from build123d import *

# Parameters (mm, degrees)
PAD017_DEPTH    = 28
SKETCH059_R     = 1.3
POCKET008_DEPTH = 48


with BuildPart() as part:
    # Sketch055 → Pad017 (new body)
    with BuildSketch(Plane.YZ):
        with BuildLine():
            ThreePointArc((0, -20.4), (17.463482, -10.544515), (18.053328, 9.499334))
            Line((18.053328, 9.499334), (23.529825, 12.66119))
            ThreePointArc((0, -26.72), (22.937583, -13.704952), (23.529825, 12.66119))
            Line((0, -20.4), (0, -26.72))
        make_face()
    extrude(amount=-PAD017_DEPTH)

    # Sketch056 → AdditiveLoft002 section 0
    with BuildSketch(Plane.YZ):
        with BuildLine():
            Line((19.650206, 5.479909), (25.72, 5.479909))
            Line((25.72, 5.479909), (25.72, -5.479909))
            Line((25.72, -5.479909), (19.650206, -5.479909))
            ThreePointArc((19.650206, -5.479909), (20.4, 0), (19.650206, 5.479909))
        make_face()
    # Sketch057 → AdditiveLoft002 section 1
    with BuildSketch(Plane.YZ.offset(17.36)):
        with BuildLine():
            Line((19.650206, 5.479909), (23.06, 5.479909))
            Line((23.06, 5.479909), (23.06, -5.479909))
            Line((23.06, -5.479909), (19.650206, -5.479909))
            ThreePointArc((19.650206, -5.479909), (20.4, 0), (19.650206, 5.479909))
        make_face()
    loft()

    # Sketch058 → Groove001 (revolve, cut)
    with BuildSketch(Plane.XY):
        Polygon((-28, 27.4), (-26, 27.4), (-26, 25.4), (-4, 25.4), (0, 27.709401), (0, 63.2), (-28, 63.2), align=None)
    revolve(axis=Axis((0, 0, 0), (1, 0, 0)), mode=Mode.SUBTRACT)

    # Sketch059 → Pocket008 (cut)
    with BuildSketch(Plane.YZ.offset(20.4)):
        with Locations((22.695, 0)):
            Circle(SKETCH059_R)
    extrude(amount=-POCKET008_DEPTH, mode=Mode.SUBTRACT)


solid = part.part
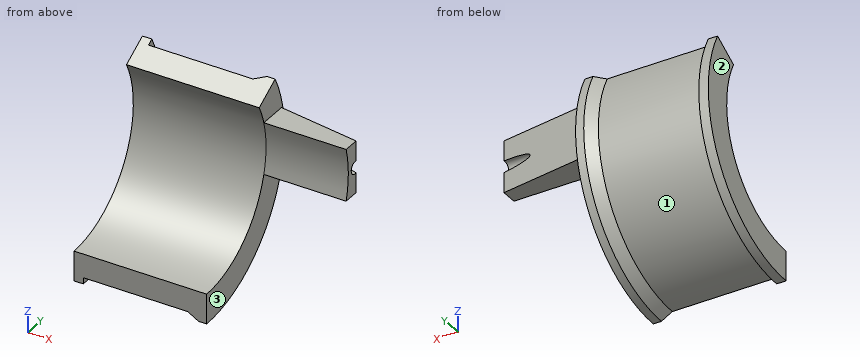
Design review of the part built by this model. Coordinates are the model's own, in mm. Face numbers are marked on the shaded views. Coordinates: 2 decimals unless noted, no trailing zeros. Loops run counter-clockwise (first coordinate to the right, second up) from the corner with the lowest first, then second, coordinate; pieces in that order, holes last. Notation, with made-up numbers: (-29, 21.25) -> (9, 21.25) arc R20 ccw to (9, 38.25) -> close; hole circle Ø7 at (59.5, 81.25). An arc over 180 degrees is marked (long way). Use a Markdown table: item, result. Add a question column.
Item 1: The part is to be moulded in two halves that separate along X. For the marked faces 1, 2 and 3, say which applies: +X half, -X half, draft (parallel to the pull), parting line (faces both ways), or undercut.
Item 2: Clearance check with flat-ended pins moving along their axes: P1, Ø5, axis at x = -0.5, y = 6, coming from the -Z side; P2, Ø10, axis at x = -2.5, y = 18.5, coming from the -Z side; P3, Ø3, axis at x = -6.5, z = 8.5, coming from the +Y side. State where each tip first meets the part, or that it passes through.
Item 3: Wall thickness on L1, parallel to Z at x = -4.5, y = 18.75; L2, parallel to X at y = 20.5, z = -13; L3, parallel to Z at x = -12.5, y = 3: over which ranges is each line inside the solid? List them lowest first. Write a range as from..to.
Item 4: We need section A-A, the plane z = 0. Write out the cut boundary in (x, y) (3 decimals), and give its area (3 significant figures).
Item 5: We need section B-B, the plane x = -12. Write out the cut boundary in (y, z) (3 decimals).
Numbers:
| question | item | result |
|---|---|---|
| 1 | face 1 | undercut |
| 1 | face 2 | -X half |
| 1 | face 3 | +X half |
| 2 | P1 | stops at z = -26.49 |
| 2 | P2 | stops at z = -23.02 |
| 2 | P3 | stops at y = 24.42 |
| 3 | L1 | z = -17.13..-8.04, 8.04..9.9 |
| 3 | L2 | x = -28..0 |
| 3 | L3 | z = -25.22..-20.18 |
| 4 | outline | (-28, 20.4) -> (17.36, 20.4) -> (17.36, 21.395) -> (-27.6, 21.395) -> (-27.6, 23.995) -> (11.258, 23.995) -> (0, 25.72) -> (0, 26.72) -> (-1.714, 26.72) -> (-4, 25.4) -> (-26, 25.4) -> (-26, 26.72) -> (-28, 26.72) -> close |
| 4 | area | 102 mm^2 |
| 5 | outline | (0, -25.4) arc R25.4 ccw to (22.386, 12.001) -> (18.053, 9.499) arc R20.4 cw to (0, -20.4) -> close; hole circle Ø2.6 at (22.695, 0) |
